Could you check a few things on this model? Use its own coordinates, in mm. A direction names the side the tool comes from. Give positions to 0.01 mm unless a question says otherwise; leave off trailing zeros. Order: outer loops, then holes, each group sorted by start corner. A loop starts at its lowest first (then second) coordinate and runs counter-clockwise, first axis right, second up. Notation, with made-up numbers: (21.25, -28) -> (30.25, -28) arc R22 cw to (30.25, -7) -> close; hole circle Ø5 at (60, 0). An arc over 180 degrees is marked (long way). Use one line per item in the form item = value. Start each with the question number.
from build123d import *

# Parameters (mm, degrees)
SKETCH1_R               = 0.5
BOSS_EXTRUDE1_DEPTH     = 4.8
SKETCH3_W               = 11.720240581
SKETCH3_H               = 3.048700617
SKETCH3_W_2             = 11.288820682
SKETCH3_H_2             = 3.839637098
CUT_EXTRUDE1_DEPTH      = 6.889299393
CUT_EXTRUDE1_DEPTH_BACK = 6.889299393


with BuildPart() as part:
    # Sketch1 → Boss-Extrude1 (new body, symmetric)
    with BuildSketch(Plane(origin=(0, 0, 0), x_dir=(1, 0, 0), z_dir=(0, 1, 0))):
        with BuildLine():
            Line((-3, 9), (-3, -1.091261391))
            Line((-3, -1.091261391), (-5.78345363, -6.64968985))
            ThreePointArc((-5.78345363, -6.64968985), (-5.88797422, -7.148913405), (-5.732690839, -7.634748546))
            Line((-5.732690839, -7.634748546), (-5.5, -8))
            ThreePointArc((-5.5, -8), (0, -6.665364504), (5.5, -8))
            Line((5.5, -8), (5.732690839, -7.634748546))
            ThreePointArc((5.732690839, -7.634748546), (5.88797422, -7.148913405), (5.78345363, -6.64968985))
            Line((5.78345363, -6.64968985), (3, -1.091261391))
            Line((3, -1.091261391), (3, 9))
            ThreePointArc((3, 9), (0, 12), (-3, 9))
        make_face()
        with Locations((0, -1.22)):
            Circle(SKETCH1_R, mode=Mode.SUBTRACT)
    extrude(amount=BOSS_EXTRUDE1_DEPTH, both=True)

    # Sketch3 → Cut-Extrude1 (cut, two sides)
    with BuildSketch(Plane(origin=(0, 0, 0), x_dir=(0, 0, -1), z_dir=(1, 0, 0))) as cut_extrude1_sk:
        with Locations((-4.389443778, 4.624350309)):
            Rectangle(SKETCH3_W, SKETCH3_H)
        with Locations((-4.173733829, -5.019818549)):
            Rectangle(SKETCH3_W_2, SKETCH3_H_2)
    extrude(amount=CUT_EXTRUDE1_DEPTH, mode=Mode.SUBTRACT)
    extrude(cut_extrude1_sk.sketch, amount=-CUT_EXTRUDE1_DEPTH_BACK, mode=Mode.SUBTRACT)


solid = part.part
(1) Imagine slicing it at A-A (x = 0). Write out the boundary of the cut face in (y, z).
(2) We'd pull the mould along X, two halves only. Please class faces 1 (the cylindrical face through (-0.108, -0.043, 1.708)), 2 (the flat face through (0, 3.1, 3)), 3 (the flat face through (-3, 0, -4)): pulls with the +X half, pulls with the -X half, needs draft (parallel to the pull), parting line crosses it, or undercut.
(3) Imagine slicing it at C-C (z = -2). Write out the boundary of the cut face in (x, y).
(4) I'm going to push flat-ended pins straight in: pin 1 Ø3 at (x, y) = (-2, 1.5) entering from +Z; pin 2 Ø3 at (x, z) = (-2, 1) entering from +Y; pin 3 Ø5 at (y, z) = (-1, -6) entering from +X; pin 4 Ø1.5 at (x, z) = (-4.5, -6.5) entering from -Y. Where does each tip first touch, or does it pass through?
(5) Please list where these lines run through material, in increasing order: probe 1 along Z at (x, y) = (0, -1.5); probe 2 along X at (y, z) = (-4.5, -2.75); probe 3 along Y at (x, z) = (0, 3).
(6) Imagine slicing it at D-D (y = -3.5). Write out the boundary of the cut face in (x, z).
(7) Imagine slicing it at B-B (y = -2.5). Write out the boundary of the cut face in (x, z).
(8) Which directions (+Z, -Z, +X, -X, +Y, -Y) give clear straight access to the entire face, cutting with the end or side of a thin tool? Please do faces 4 (the flat face through (0, 4, -1.471)), 5 (the flat face through (-4.37, 0.04, 3.83)), 6 (the flat face through (0, -3.1, 3)), 7 (the flat face through (3, 0, -4)).
Calculated:
q1.outline = (-4.8, -12) -> (4.8, -12) -> (4.8, -1.47) -> (3.1, -1.47) -> (3.1, 0.72) -> (-3.1, 0.72) -> (-3.1, -1.47) -> (-4.8, -1.47) -> close; (-3.1, 1.72) -> (3.1, 1.72) -> (3.1, 6.67) -> (-3.1, 6.67) -> close
q2.face_1 = undercut
q2.face_2 = needs draft
q2.face_3 = pulls with the -X half
q3.outline = (-3, -4.8) -> (3, -4.8) -> (3, 4.8) -> (-3, 4.8) -> close
q4.pin_1 = 7.19
q4.pin_2 = 3.1
q4.pin_3 = 3
q4.pin_4 = through
q5.probe_1 = -12 to 0.72, 1.72 to 6.67
q5.probe_2 = -3 to 3
q5.probe_3 = -3.1 to 3.1
q6.outline = (-3, -9) arc R3 ccw to (3, -9) -> (3, -1.47) -> (-3, -1.47) -> close
q7.outline = (-5.78, 6.65) -> (-3, 1.09) -> (-3, -9) arc R3 ccw to (3, -9) -> (3, 1.09) -> (5.78, 6.65) arc R1 ccw to (5.73, 7.63) -> (5.5, 8) arc R12 cw to (-5.5, 8) -> (-5.73, 7.63) arc R1 ccw to start; hole circle Ø1 at (0, 1.22)
q8.face_4 = +Z, +X, -X, +Y
q8.face_5 = -Z, -X, +Y, -Y
q8.face_6 = +Z, +X, -X, -Y
q8.face_7 = -Z, +X, +Y, -Y
